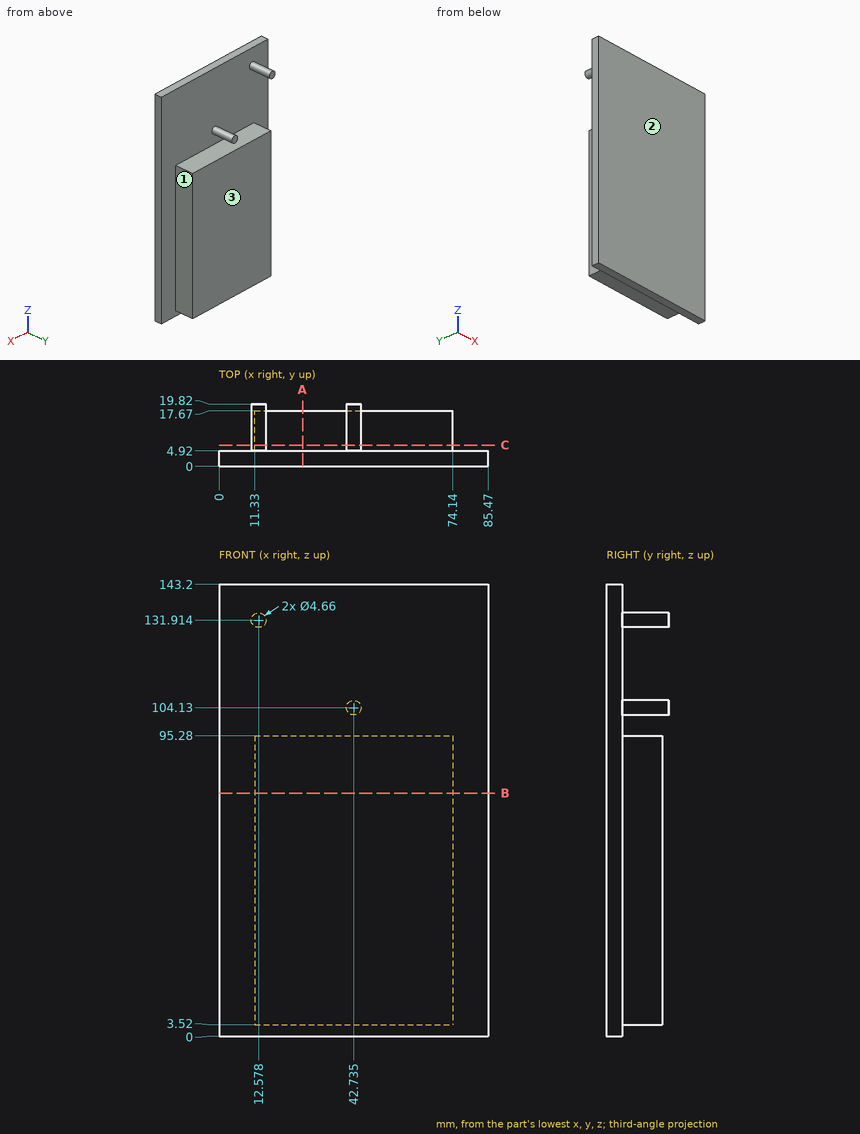
Answer from the drawing. Dimensions are ordinates in mm from the lowest x, y and z of the part. A direction names the side the tool comes from. Give positions to 0.01 mm unless a question says otherwise; leave off trailing zeros. Order: outer loops, then holes, each group sorted by start corner. A loop starts at its lowest first (then second) coordinate and runs counter-clockwise, first axis right, second up. Notation, with made-up numbers: (34.5, 11) - (41.5, 11) arc R9 ccw to (41.5, 21) - close; hole circle Ø8 at (-7.5, 21.25). An arc over 180 degrees is marked (long way). One line per item, written item: value. Start each with the question number.
1. Each of these flat-tipped pins is pushed along its axis until it touches: pin 1 Ø2 at (x, y) = (21.5, 6.5) entering from -Z; pin 2 Ø10 at (x, y) = (29, 17) entering from +Z; pin 3 Ø2 at (y, z) = (7.5, 28) entering from -X. Where does it stop, or does it pass through?
2. Section A-A, the plane x = 26.5 is taken. Write down the section's boundary in (y, z), then the cut area to 3 significant figures.
3. Which of the six approach directions +Z, -Z, +X, -X, +Y, -Y give full straight-line access (tool end or side, diameter ignored) to the marked faces 1, 2 and 3?
4. Section B-B, the plane z = 77 is taken. Write down the section's boundary in (x, y).
5. Consider line 1 (Y direction, x = 48.5, z = 76.5); line 2 (X direction, y = 17.5, z = 16); line 3 (Z direction, x = 50, y = 11.75). Determine where each line is inside the solid, lowest interval first.
6. Section C-C, the plane y = 6.75 is taken. Write down the section's boundary in (x, z) (3 decimals), then the cut area to 3 significant figures.
Filled sheet:
1. pin 1: z = 3.52
1. pin 2: z = 95.28
1. pin 3: x = 11.33
2. outline: (0, 0) - (4.92, 0) - (4.92, 3.52) - (17.67, 3.52) - (17.67, 95.28) - (4.92, 95.28) - (4.92, 143.2) - (0, 143.2) - close
2. area: 1,870 mm²
3. face 1: +Z, -Z, +X, +Y
3. face 2: +Z, -Z, +X, -X, -Y
3. face 3: -Z, +X, -X, +Y
4. outline: (0, 0) - (85.47, 0) - (85.47, 4.92) - (74.14, 4.92) - (74.14, 17.67) - (11.33, 17.67) - (11.33, 4.92) - (0, 4.92) - close
5. line 1: 0 to 17.67
5. line 2: 11.33 to 74.14
5. line 3: 3.52 to 95.28
6. outline: circle Ø4.66 at (12.578, 131.914); (11.33, 3.52) - (74.14, 3.52) - (74.14, 95.28) - (11.33, 95.28) - close; circle Ø4.66 at (42.735, 104.13)
6. area: 5,800 mm²
